from build123d import *

# Parameters (mm, degrees)
F0_R      = 30
F1_DEPTH  = 20
F2_R      = 21.9
F3_DEPTH  = 3
F4_R      = 21.9
F5_DEPTH  = 2
F6_SIZE   = 2
F7_R      = 20
F8_DEPTH  = 45
F9_R      = 21.9
F10_DEPTH = 3
F12_DEPTH = 86.2
F14_DEPTH = 70
F16_DEPTH = 60.5


with BuildPart() as f1:
    # F0 (on Top) → F1 (new body)
    with BuildSketch(Plane.XY):
        Circle(F0_R)
    extrude(amount=F1_DEPTH)

    # F2 (on face) → F3 (join)
    with BuildSketch(Plane.XY.offset(20)):
        Circle(F2_R)
    extrude(amount=F3_DEPTH)

    # F4 (on face) → F5 (join)
    with BuildSketch(Plane.XY.offset(23)):
        Circle(F4_R)
    extrude(amount=F5_DEPTH)

    # F6
    f6_edges = [f1.edges().sort_by_distance(p)[0] for p in [
        (-21.9, 0, 25),
    ]]
    chamfer(f6_edges, length=F6_SIZE)

    # F7 (on face) → F8 (join)
    with BuildSketch(Plane.XY.offset(25)):
        Circle(F7_R)
    extrude(amount=F8_DEPTH)

    # F9 (on face) → F10 (join)
    with BuildSketch(Plane.XY.offset(70)):
        Circle(F9_R)
    extrude(amount=F10_DEPTH)

    # F11 (on face) → F12 (cut)
    with BuildSketch(Plane.XY.offset(73)):
        with BuildLine():
            Line((-15, 0), (15, 0))
            ThreePointArc((15, 0), (14.8635877974, 2.0183552187), (14.4568322948, 4))
            ThreePointArc((14.4568322948, 4), (-2.0183552187, 14.8635877974), (-15, 0))
        make_face()
        with BuildLine():
            Line((18, 0), (15, 0))
            ThreePointArc((15, 0), (14.8635877974, -2.0183552187), (14.4568322948, -4))
            Line((14.4568322948, -4), (18, -4))
            Line((18, -4), (18, 0))
        make_face()
        with BuildLine():
            ThreePointArc((14.4568322948, -4), (14.8635877974, -2.0183552187), (15, 0))
            Line((15, 0), (-15, 0))
            ThreePointArc((-15, 0), (-2.0183552187, -14.8635877974), (14.4568322948, -4))
        make_face()
        with BuildLine():
            ThreePointArc((14.4568322948, 4), (14.8635877974, 2.0183552187), (15, 0))
            Line((15, 0), (18, 0))
            Line((18, 0), (18, 4))
            Line((18, 4), (14.4568322948, 4))
        make_face()
    extrude(amount=-F12_DEPTH, mode=Mode.SUBTRACT)

    # F13 (on Front) → F14 (cut)
    with BuildSketch(Plane.XZ):
        with BuildLine():
            ThreePointArc((0, 6), (2.8284271247, 7.1715728753), (4, 10))
            ThreePointArc((4, 10), (-2.8284271247, 12.8284271247), (0, 6))
        make_face()
    extrude(amount=F14_DEPTH, mode=Mode.SUBTRACT)

    # F15 (on Right) → F16 (cut)
    with BuildSketch(Plane.YZ):
        with BuildLine():
            ThreePointArc((0, 6), (2.8284271247, 7.1715728753), (4, 10))
            ThreePointArc((4, 10), (-2.8284271247, 12.8284271247), (0, 6))
        make_face()
    extrude(amount=F16_DEPTH, mode=Mode.SUBTRACT)


solid = f1.part
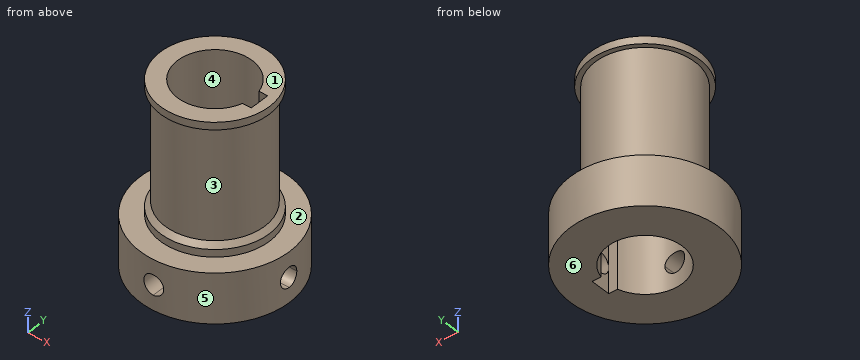
For this review, take the finished solid that the model builds, in its own axes (mm). Face numbers are marked on the shaded views. A direction names the side the tool comes from. Round coordinates to 2 decimals unless told otherwise and drop trailing zeros. Order: outer loops, then holes, each group sorted by start corner. A loop starts at its lowest first (then second) coordinate and runs counter-clockwise, first axis right, second up. Notation, with made-up numbers: M 89.5,33.25 L 114.5,33.25 A19 ccw 114.5,51.25 Z; hole C -28,7.25 d1. An arc over 180 degrees is marked long. Use a Markdown table: item, result. Add a question column.
Item 1: Add section B-B, the plane x = 24. Give the boundary of the cut face in (y, z).
Item 2: To check wall thickness, follow line 1 along Z through (x, y) = (19.5, 22); line 2 along Z through (x, y) = (27, 0); line 3 along Z through (x, y) = (0, -21.25). State the ranges of each line that lie inside material, in increasing order.
Item 3: Mouldability with a two-part tool opening along X and no side actions: class the marked faces 4, 5 and 6 as released by +X, released by -X, zero draft, split by the parting line, or undercut.
Item 4: Add section A-A, the plane z = 19. Give the boundary of the cut face in (x, y), then the cut area to 3 significant figures.
Item 5: Add section C-C, the plane z = 54.5. Give the boundary of the cut face in (x, y), then the cut area to 3 significant figures.
Item 6: Add section D-D, the plane x = -3. State how many separate pieces and enclosed holes the cut face has, then the cut area to 3 significant figures.
Item 7: Tool access review of the marked faces 1, 2 and 3: name each direction out of +Z, -Z, +X, -X, +Y, -Y from which nothing blocks a thin tool from reaching the whole face with its end or side.
Item 8: Insertion check: pin 1 (5 mm diameter, centred on x = 11.5, z = 51, fed in from -Y); pin 2 (3 mm diameter, centred on y = 3.5, z = 59.5, fed in from +X); pin 3 (9 mm diameter, centred on x = 0, z = 10, fed in from -Y); pin 4 (4 mm diameter, centred on x = 16.5, z = 45, fed in from +Y) (3 decimals). Each pin has a flat end and moves straight along its axis. Give the tip position at first contact, or say it passes through.
Geometry results:
| question | item | result |
|---|---|---|
| 1 | outline | M -18,0 L 18,0 L 18,20 L -18,20 Z; hole C 0,10 d8 |
| 2 | line 1 | z = 0 to 20 |
| 2 | line 2 | z = 0 to 6, 14 to 20 |
| 2 | line 3 | z = 0 to 6, 14 to 23.65, 70 to 73 |
| 3 | face 4 | undercut |
| 3 | face 5 | split by the parting line |
| 3 | face 6 | zero draft |
| 4 | outline | C 0,0 d60; hole M 14.46,-4 L 18,-4 L 18,4 L 14.46,4 A15 ccw long Z |
| 4 | area | 2,100 mm² |
| 5 | outline | C 0,0 d40; hole M 14.46,-4 L 18,-4 L 18,4 L 14.46,4 A15 ccw long Z |
| 5 | area | 524 mm² |
| 6 | separate pieces | 3 |
| 6 | enclosed holes | 0 |
| 6 | area | 1,090 mm² |
| 7 | face 1 | +Z, +X, -X, +Y, -Y |
| 7 | face 2 | +Z |
| 7 | face 3 | none |
| 8 | pin 1 | stops at y = -17.86 |
| 8 | pin 2 | stops at x = 19.9 |
| 8 | pin 3 | stops at y = -30 |
| 8 | pin 4 | stops at y = 13.775 |
